Verification items for the finished model (mm, model axes). A direction names the side the tool comes from. Round coordinates to 2 decimals unless told otherwise and drop trailing zeros. Order: outer loops, then holes, each group sorted by start corner. A loop starts at its lowest first (then second) coordinate and runs counter-clockwise, first axis right, second up. Notation, with made-up numbers: M -14,52 L 29,52 A27 ccw 29,81 Z; hole C 73.5,1.5 d3. An arc over 180 degrees is marked long. One line per item, written item: value. Start each with the question number.
from build123d import *

# Parameters (mm, degrees)
SKETCH3_W           = 31.75
SKETCH3_H           = 67.207500078
SKETCH3_R           = 2.200000045
BOSS_EXTRUDE1_DEPTH = 6.35
SKETCH5_W           = 31.75
SKETCH5_H           = 6.35
BOSS_EXTRUDE2_DEPTH = 50.8
SKETCH6_R           = 1.777000002
CUT_EXTRUDE1_DEPTH  = 7.35
CUT_EXTRUDE2_DEPTH  = 51.8


with BuildPart() as part:
    # Sketch3 → Boss-Extrude1 (new body)
    with BuildSketch(Plane(origin=(0, 0, 0), x_dir=(0, 0, -1), z_dir=(1, 0, 0))):
        with Locations((15.875, 33.603750039)):
            Rectangle(SKETCH3_W, SKETCH3_H)
        with Locations((10.874999967, 8.935000037)):
            Circle(SKETCH3_R, mode=Mode.SUBTRACT)
        with Locations((20.875000033, 8.935000037)):
            Circle(SKETCH3_R, mode=Mode.SUBTRACT)
        with Locations((10.874999967, 57.535000119)):
            Circle(SKETCH3_R, mode=Mode.SUBTRACT)
        with Locations((20.875000033, 57.535000119)):
            Circle(SKETCH3_R, mode=Mode.SUBTRACT)
        Polygon((5.748000061, 54.507500078), (14.875, 54.507500078), (14.875, 61.111500078), (16.875, 61.111500078), (16.875, 54.507500078), (26.001999939, 54.507500078), (26.001999939, 11.962500078), (16.875, 11.962500078), (16.875, 5.358500078), (14.875, 5.358500078), (14.875, 11.962500078), (5.748000061, 11.962500078), align=None, mode=Mode.SUBTRACT)
    extrude(amount=BOSS_EXTRUDE1_DEPTH)

    # Sketch5 → Boss-Extrude2 (add)
    with BuildSketch(Plane(origin=(6.35, 0, 0), x_dir=(0, 0, -1), z_dir=(1, 0, 0))):
        with Locations((15.875, -3.175)):
            Rectangle(SKETCH5_W, SKETCH5_H)
    extrude(amount=-BOSS_EXTRUDE2_DEPTH)

    # Sketch6 → Cut-Extrude1 (cut, through all)
    with BuildSketch(Plane(origin=(0, 0, 0), x_dir=(1, 0, 0), z_dir=(0, 1, 0))):
        with Locations((-6.35, 6.35)):
            Circle(SKETCH6_R)
        with Locations((-38.1, 15.875)):
            Circle(SKETCH6_R)
        with Locations((-6.35, 25.4)):
            Circle(SKETCH6_R)
    extrude(amount=-CUT_EXTRUDE1_DEPTH, mode=Mode.SUBTRACT)

    # Sketch7 → Cut-Extrude2 (cut, through all)
    with BuildSketch(Plane(origin=(6.35, 0, 0), x_dir=(0, 0, -1), z_dir=(1, 0, 0))):
        with BuildLine():
            Line((0, 61.774194579), (0, 82.748877538))
            Line((0, 82.748877538), (31.75, 82.748877538))
            Line((31.75, 82.748877538), (31.75, 61.774194579))
            ThreePointArc((31.75, 61.774194579), (15.875, 65.0875), (0, 61.774194579))
        make_face()
    extrude(amount=-CUT_EXTRUDE2_DEPTH, mode=Mode.SUBTRACT)


solid = part.part
1. Draft check along Y on faces 3 (the face through (0, 33, -5)), 4 (the face through (3, 58, -16.875)), 5 (the face through (-19, -6.35, -16)). Enter one of: released by +Y, released by -Y, zero draft, split by the parting line, or undercut.
2. Scan lines: line 1 along Z through (x, y) = (2.5, 28); line 2 along Y through (x, z) = (-11.5, -18); line 3 along X through (y, z) = (57, -8). Record each from-to range of solid material in increasing order.
3. Depth check by flat-ended pin: pin 1 (5 mm diameter, centred on y = 8.935, z = -10.875, fed in from -X); pin 2 (4 mm diameter, centred on x = -38.1, z = -15.875, fed in from +Y); pin 3 (3 mm diameter, centred on x = 3.5, z = -22, fed in from +Y). Enter the tip coordinate at first touch or a pass-through.
4. Section check A-A (y = 23). Record the cut outline in (x, z), and give its area (3 significant figures).
5. Section check D-D (x = -6.35). Record the cut outline in (y, z).
6. Section check C-C (z = -11.5). Record the cut outline in (x, y).
7. Tool access check on faces 1 (the face through (-6.735, -3.131, -23.665)), 2 (the face through (3, 9, -16.875)). Record the directions out of +Z, -Z, +X, -X, +Y, -Y that give a thin tool (end or side, any length) a straight path to the whole face; none if there is none.
8. Section check B-B (x = -38.1). Record the cut outline in (y, z), and give its area (3 significant figures).
Geometry check:
1. face 3: zero draft
1. face 4: undercut
1. face 5: released by -Y
2. line 1: z = -31.75 to -26, -5.75 to 0
2. line 2: y = -6.35 to 0
2. line 3: x = 0 to 6.35
3. pin 1: stops at x = 0
3. pin 2: stops at y = 0
3. pin 3: stops at y = 64.82
4. outline: M 0,-31.75 L 6.35,-31.75 L 6.35,-26 L 0,-26 Z; M 0,-5.75 L 6.35,-5.75 L 6.35,0 L 0,0 Z
4. area: 73.0 mm²
5. outline: M -6.35,-31.75 L 0,-31.75 L 0,-27.18 L -6.35,-27.18 Z; M -6.35,-23.62 L 0,-23.62 L 0,-8.13 L -6.35,-8.13 Z; M -6.35,-4.57 L 0,-4.57 L 0,0 L -6.35,0 Z
6. outline: M -44.45,-6.35 L 6.35,-6.35 L 6.35,6.83 L 0,6.83 L 0,0 L -44.45,0 Z; M 0,11.04 L 6.35,11.04 L 6.35,11.96 L 0,11.96 Z; M 0,54.51 L 6.35,54.51 L 6.35,55.43 L 0,55.43 Z; M 0,59.64 L 6.35,59.64 L 6.35,64.85 L 0,64.85 Z
7. face 1: +Y, -Y
7. face 2: +X, -X
8. outline: M -6.35,-31.75 L 0,-31.75 L 0,-17.65 L -6.35,-17.65 Z; M -6.35,-14.1 L 0,-14.1 L 0,0 L -6.35,0 Z
8. area: 179 mm²
